Geometry check sheet. Reference: drawing and pictorial views, mm from the part's lowest x, y, z. A direction names the side the tool comes from. Round coordinates to 2 decimals unless told otherwise and drop trailing zeros. Loops run counter-clockwise (first coordinate to the right, second up) from the corner with the lowest first, then second, coordinate; pieces in that order, holes last. Notation, with made-up numbers: (-25.5, 19) -> (-8.5, 19) arc R7 cw to (-8.5, 28) -> close; hole circle Ø5 at (-5, -30.5). An arc over 180 degrees is marked (long way). Use one line per item in the form item = value.
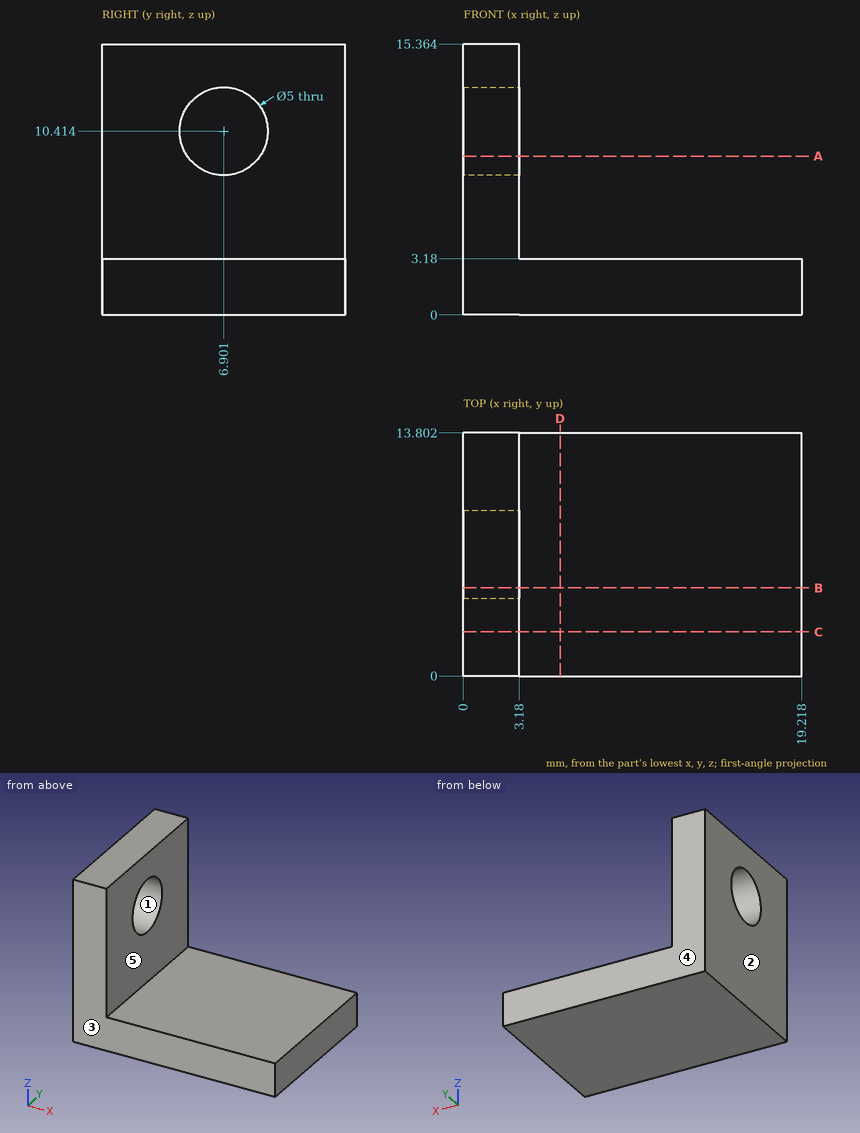
1. Tool access check on the marked faces 4 and 5. Record the directions out of +Z, -Z, +X, -X, +Y, -Y that give a thin tool (end or side, any length) a straight path to the whole face; none if there is none.
Return value:
face_4 = +Z, -Z, +X, -X, +Y
face_5 = +Z, +X, +Y, -Y
2. Section check B-B (y = 5). Record the boundary of the cut face in (x, z).
Return value:
outline = (0, 0) -> (19.22, 0) -> (19.22, 3.18) -> (3.18, 3.18) -> (3.18, 8.79) -> (0, 8.79) -> close; (0, 12.04) -> (3.18, 12.04) -> (3.18, 15.36) -> (0, 15.36) -> close
3. Material ranges on line 1 along X through (y, z) = (2.75, 12); line 2 along Z through (x, y) = (1, 7.25), recorded low to high.
Return value:
line_1 = 0 to 3.18
line_2 = 0 to 7.94, 12.89 to 15.36
4. Gauge pin test, flat ends, axial feed: pin 1 (8 mm diameter, centred on y = 6.9, z = 10.41, fed in from +X); pin 2 (7 mm diameter, centred on x = 10.5, y = 4.5, fed in from +Z). Record the tip position at first contact, or that the pin passes through.
Return value:
pin_1 = 3.18
pin_2 = 3.18
5. Section check A-A (z = 9). Record the boundary of the cut face in (x, y).
Return value:
outline = (0, 0) -> (3.18, 0) -> (3.18, 4.84) -> (0, 4.84) -> close; (0, 8.96) -> (3.18, 8.96) -> (3.18, 13.8) -> (0, 13.8) -> close
6. Section check D-D (x = 5.5). Record the boundary of the cut face in (y, z).
Return value:
outline = (0, 0) -> (13.8, 0) -> (13.8, 3.18) -> (0, 3.18) -> close
7. Section check C-C (y = 2.5). Record the boundary of the cut face in (x, z).
Return value:
outline = (0, 0) -> (19.22, 0) -> (19.22, 3.18) -> (3.18, 3.18) -> (3.18, 15.36) -> (0, 15.36) -> close
8. Mould release check, pull along Y, two halves, no side actions. Record for the marked faces 1, 2 and 3: released by +Y, released by -Y, zero draft, split by the parting line, or undercut.
Return value:
face_1 = undercut
face_2 = zero draft
face_3 = released by -Y
